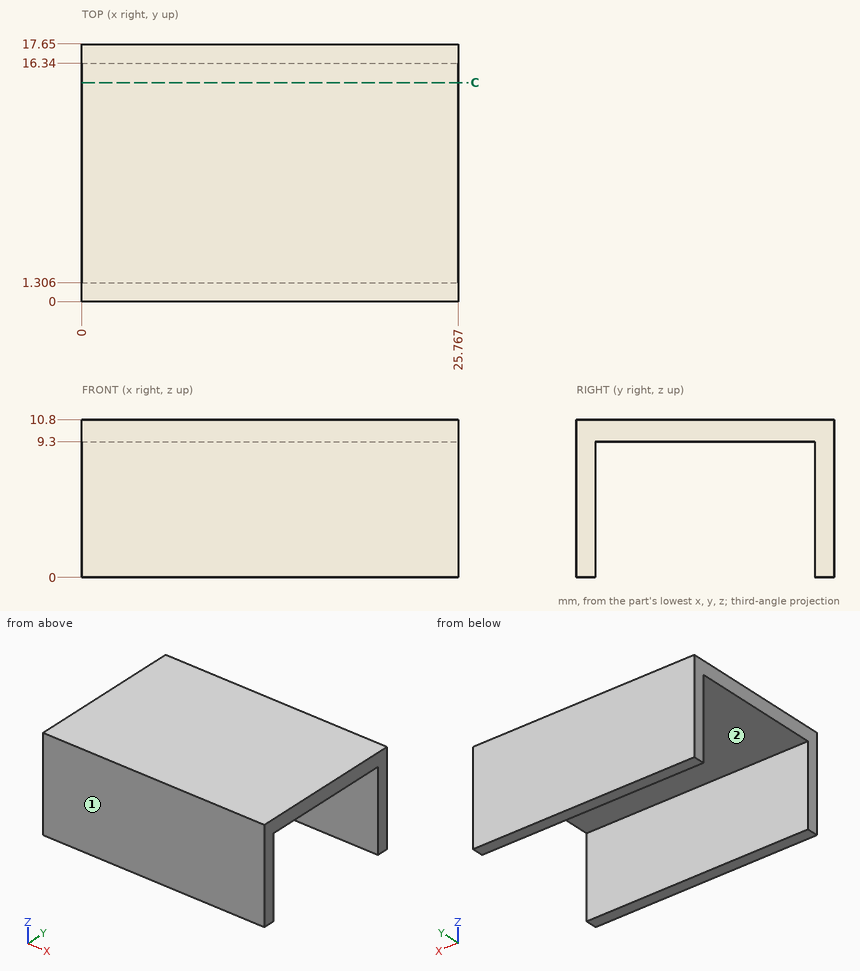
For this review, use the dimensioned drawing (mm, ordinates from the lowest corner) and the shaded views. A direction names the side the tool comes from. Round coordinates to 2 decimals unless told otherwise and drop trailing zeros. Order: outer loops, then holes, each group sorted by start corner. A loop starts at its lowest first (then second) coordinate and runs counter-clockwise, first axis right, second up. Notation, with made-up numbers: (76, -4.5) - (121, -4.5) arc R10 ccw to (121, 7.5) - close; hole circle Ø4 at (-25.5, 69). An arc over 180 degrees is marked (long way). Use one line per item in the form item = value.
Q1. Tool access review of the marked faces 1 and 2: name each direction out of +Z, -Z, +X, -X, +Y, -Y from which nothing blocks a thin tool from reaching the whole face with its end or side.
Response values:
face_1 = +Z, -Z, +X, -X, -Y
face_2 = -Z, +X, -X
Q2. To check wall thickness, follow line 1 (Z direction, x = 13.25, y = 1.5). State the ranges of the line that lie inside material, in increasing order.
Response values:
line_1 = 9.3 to 10.8
Q3. Add section C-C on y = 15. Give the boundary of the cut face in (x, z).
Response values:
outline = (0, 9.3) - (25.77, 9.3) - (25.77, 10.8) - (0, 10.8) - close
Q4. Clearance check with a flat-ended pin moving along its axis: P1, Ø3, axis at x = 18, y = 9, coming from the -Z side. State where the tip first meets the part, or that it passes through.
Response values:
P1 = 9.3
